Geometry check sheet. Reference: the model listing, model coordinates, mm. Face numbers are marked on the shaded views. A direction names the side the tool comes from. Round coordinates to 2 decimals unless told otherwise and drop trailing zeros. Order: outer loops, then holes, each group sorted by start corner. A loop starts at its lowest first (then second) coordinate and runs counter-clockwise, first axis right, second up.
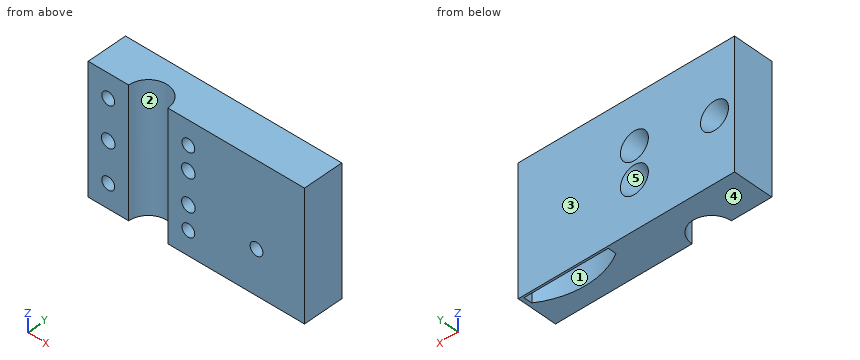
```python
from build123d import *

# Parameters (mm, degrees)
SKETCH056_W     = 30
SKETCH056_H     = 32
SKETCH056_R     = 1.7
PAD037_DEPTH    = 10
SKETCH057_R     = 3.5
POCKET020_DEPTH = 5
POCKET020_TAPER = 20
SKETCH059_R     = 4.9
POCKET022_DEPTH = 32
SKETCH060_W     = 32
SKETCH060_H     = 10
PAD038_DEPTH    = 24
POCKET023_DEPTH = 28
SKETCH062_R     = 1.6
POCKET024_DEPTH = 8


with BuildPart() as part:
    # Sketch056 → Pad037 (new body)
    with BuildSketch(Plane.XZ):
        Rectangle(SKETCH056_W, SKETCH056_H)
        with Locations((10, 4)):
            Circle(SKETCH056_R, mode=Mode.SUBTRACT)
        with Locations((10, -4)):
            Circle(SKETCH056_R, mode=Mode.SUBTRACT)
        with Locations((-10, 0)):
            Circle(SKETCH056_R, mode=Mode.SUBTRACT)
    extrude(amount=PAD037_DEPTH)

    # Sketch057 (on Face8 of Pad037) → Pocket020 (cut)
    with BuildSketch(Plane(origin=(0, 0, 0), x_dir=(1, 0, 0), z_dir=(0, 1, 0))):
        with Locations((-10, 0)):
            Circle(SKETCH057_R)
        with Locations((10, 4)):
            Circle(SKETCH057_R)
        with Locations((10, -4)):
            Circle(SKETCH057_R)
    extrude(amount=-POCKET020_DEPTH, taper=POCKET020_TAPER, mode=Mode.SUBTRACT)

    # Sketch059 (on Face1 of Pocket020) → Pocket022 (cut)
    with BuildSketch(Plane(origin=(0, 0, -16), x_dir=(1, 0, 0), z_dir=(0, 0, -1))):
        with Locations((0, 10)):
            Circle(SKETCH059_R)
    extrude(amount=-POCKET022_DEPTH, mode=Mode.SUBTRACT)

    # Sketch060 (on Face3 of Pocket022) → Pad038 (join)
    with BuildSketch(Plane(origin=(15, 0, 0), x_dir=(0, 0, 1), z_dir=(1, 0, 0))):
        with Locations((0, 5)):
            Rectangle(SKETCH060_W, SKETCH060_H)
    extrude(amount=PAD038_DEPTH)

    # Sketch061 (on Face2 of Pad038) → Pocket023 (cut)
    with BuildSketch(Plane(origin=(0, 0, -16), x_dir=(1, 0, 0), z_dir=(0, 0, -1))):
        with BuildLine():
            Line((17, 2.6), (17, 0.5))
            Line((17, 0.5), (38, 0.5))
            Line((38, 0.5), (38, 2.6))
            ThreePointArc((38, 2.6), (27.5, 5.6), (17, 2.6))
        make_face()
    extrude(amount=-POCKET023_DEPTH, mode=Mode.SUBTRACT)

    # Sketch062 (on Face3 of Pocket023) → Pocket024 (cut)
    with BuildSketch(Plane.XZ.offset(10)):
        with Locations((-10, 10)):
            Circle(SKETCH062_R)
        with Locations((-10, -10)):
            Circle(SKETCH062_R)
        with Locations((10, 10)):
            Circle(SKETCH062_R)
        with Locations((10, -10)):
            Circle(SKETCH062_R)
        with Locations((27, -5)):
            Circle(SKETCH062_R)
    extrude(amount=-POCKET024_DEPTH, mode=Mode.SUBTRACT)


with BuildPart() as part_1:
    # Body010 placement: moved
    add(part.part.moved(Location((-1, -43.5, 39.5))))


solid = part_1.part
```
(1) Sectioned sample at B-B, the plane z = 49.5. Record the cut outline in (x, y) (3 decimals), and give its area (3 significant figures).
Returned:
outline: (-16, -53.5) - (-12.6, -53.5) - (-12.6, -45.5) - (-9.4, -45.5) - (-9.4, -53.5) - (-5.9, -53.5) arc R4.9 cw to (3.9, -53.5) - (7.4, -53.5) - (7.4, -45.5) - (10.6, -45.5) - (10.6, -53.5) - (38, -53.5) - (38, -43.5) - (-16, -43.5) - close; hole (16, -46.1) arc R19.875 ccw to (37, -46.1) - (37, -44) - (16, -44) - close
area: 364 mm2
(2) Depth check by flat-ended pin: P1, Ø3, axis at x = 9, z = 29.5, coming from the -Y side; P2, Ø5.5, axis at x = -11, z = 39.5, coming from the -Y side; P3, Ø1.5, axis at x = 25.5, y = -45.5, coming from the -Z side. Enter the tip coordinate at first touch or a pass-through.
Returned:
P1: stops at y = -45.5
P2: stops at y = -53.5
P3: stops at z = 51.5
(3) Sectioned sample at D-D, the plane x = 26. Record the cut outline in (y, z), and give its area (3 significant figures).
Returned:
outline: (-53.5, 23.5) - (-49.09, 23.5) - (-49.09, 32.9) - (-53.5, 32.9) - close; (-53.5, 36.1) - (-49.09, 36.1) - (-49.09, 51.5) - (-44, 51.5) - (-44, 23.5) - (-43.5, 23.5) - (-43.5, 55.5) - (-53.5, 55.5) - close
area: 163 mm2
(4) Sectioned sample at C-C, the plane y = -50.75. Give the number of separate pieces and of enclosed holes in the cut face, and give its area (3 significant figures).
Returned:
separate pieces: 2
enclosed holes: 8
area: 1,400 mm2
(5) Material ranges on line 1 (Z direction, x = 9, y = -51.5); line 2 (Z direction, x = -11, y = -49); line 3 (X direction, y = -46.25, z = 34.5) (3 decimals), recorded low to high.
Returned:
line 1: z = 23.5 to 27.9, 31.1 to 33.8, 37.2 to 41.8, 45.2 to 47.9, 51.1 to 55.5
line 2: z = 23.5 to 27.9, 31.1 to 37.8, 41.2 to 47.9, 51.1 to 55.5
line 3: x = -16 to 6.71, 11.29 to 16.245, 36.755 to 38
(6) Sectioned sample at A-A, the plane x = 9. Record the cut outline in (y, z), and give its area (3 significant figures).
Returned:
outline: (-53.5, 23.5) - (-43.5, 23.5) - (-43.5, 32) - (-48.45, 33.8) - (-53.5, 33.8) - (-53.5, 31.1) - (-45.5, 31.1) - (-45.5, 27.9) - (-53.5, 27.9) - close; (-53.5, 37.2) - (-48.45, 37.2) - (-43.5, 39) - (-43.5, 40) - (-48.45, 41.8) - (-53.5, 41.8) - close; (-53.5, 45.2) - (-48.45, 45.2) - (-43.5, 47) - (-43.5, 55.5) - (-53.5, 55.5) - (-53.5, 51.1) - (-45.5, 51.1) - (-45.5, 47.9) - (-53.5, 47.9) - close
area: 183 mm2
(7) Set-up check for the marked faces 1 and 2: record each of +Z, -Z, +X, -X, +Y, -Y from which the full face is reachable in a straight line by a thin tool's end or side.
Returned:
face 1: -Z
face 2: +Z, -Z, -Y
(8) Draft check along Z on the marked faces 3, 4 and 5. Enter one of: released by +Z, released by -Z, zero draft, split by the parting line, or undercut.
Returned:
face 3: zero draft
face 4: released by -Z
face 5: undercut
